Autodesk Inventor part; units mm, degrees
ref_plane "YZ Plane" through (0, 0, 0) normal (1, 0, 0) x (0, 1, 0)
ref_plane "XZ Plane" through (0, 0, 0) normal (0, 1, 0) x (-1, 0, 0)
ref_plane "XY Plane" through (0, 0, 0) normal (0, 0, 1) x (1, 0, 0)
sketch "Sketch2" plane through (0, 0, 0) normal (0, 1, 0) x (-1, 0, 0)
  line L0 (-12, 4) -> (12, 4)
  line L1 (12, 4) -> (12, -4)
  line L2 (12, -4) -> (-12, -4)
  line L3 (-12, -4) -> (-12, 4)
  point P0 (0, 0)
  point P1 (0, 4)
  point P2 (-12, 0)
  dimension "d0" = 24
  dimension "d1" = 8
extrude "Extrusion1" add sketch "Sketch2" along normal blind 3.2
sketch "Sketch3" plane through (0, 0, 0) normal (0, -1, 0) x (1, 0, 0)
  line L0 (12, 4) -> (-12, 4)
  line L1 (-12, 4) -> (-12, -4)
  line L2 (-10.4, 2.4) -> (10.4, 2.4)
  line L3 (10.4, 2.4) -> (10.4, -2.4)
  line L4 (10.4, -2.4) -> (-10.4, -2.4)
  line L5 (-10.4, -2.4) -> (-10.4, 2.4)
  circle A0 centre (-4, 4) radius 3.2569
  circle A1 centre (-4, 4) radius 2.4
  line L6 (-12, -4) -> (12, -4)
  circle A2 centre (-4, 0) radius 1.6
  line L7 (12, -4) -> (12, 4)
  line L8 (-8, 0) -> (0, 0) construction
  line L9 (0, 0) -> (8, 0) construction
  line L10 (-11.6, 3.6) -> (11.6, 3.6)
  line L11 (11.6, 3.6) -> (11.6, -3.6)
  line L12 (11.6, -3.6) -> (-11.6, -3.6)
  line L13 (-11.6, -3.6) -> (-11.6, 3.6)
  point P0 (-10.4, 0)
  point P1 (0, 2.4)
  point P2 (-4, 0)
  point P3 (0, 3.6)
  point P4 (-11.6, 0)
  dimension "d8" = 1.6
  dimension "d60" = 6.5137
  dimension "d61" = 4.8
  dimension "d62" = 1.6
  dimension "d75" = 8
  dimension "d76" = 8
  dimension "d86" = 3.2
  dimension "d89" = 8
  dimension "d95" = 0.4
  dimension "d96" = 0.4
extrude "Extrusion2" cut sketch "Sketch3" against normal blind 1.6 contours A0 A2 A1 L2 | L2 L3 L4 L5 A0 A2 | A1 L2 | L2 A1 A2 A0 | A2 A0 | A0 A2
extrude "Extrusion7" cut sketch "Sketch3" against normal blind 0.4 contours L7 L6 L1 L0 A0 L10 L13 L12 L11 | A0 L10 A1 L0 | A1 L10 L0 | L0 A1 L10 A0
fillet "Fillet1" radius 0.1 8 edges at (-12, 1.8, 4) (0, 3.2, 4) (-12, 3.2, 0) (0, 3.2, -4) (12, 3.2, 0) (12, 1.8, 4) (12, 1.8, -4) (-12, 1.8, -4)
sketch "Skizze10" plane through (0, 3.2, 0) normal (0, 1, 0) x (1, 0, 0)
  line L0 (-11.9, -3.9) -> (-11.9, 3.9)
  line L1 (-11.9, -3.9419) -> (-11.9, 3.9419) construction
  line L2 (-11.9, 3.9419) -> (11.9, 3.9419) construction
  line L3 (11.9, 3.9419) -> (11.9, -3.9419) construction
  line L4 (11.9, -3.9419) -> (-11.9, -3.9419) construction
  point P0 (0, 0)
  point P1 (0, 3.9419)
  point P2 (-11.9, 0)
  point P3 (-11.9, 0)
decal "Aufkleber1"
equation "\"d4\" = 0.333333 * lh"
equation "\"d8\" = d62"
equation "\"d60\" = tubeod"
equation "\"d61\" = kd"
equation "\"d62\" = wall"
equation "\"d75\" = lu"
equation "\"d76\" = d75"
equation "\"d86\" = pd"
equation "\"d89\" = lu"
equation "\"d95\" = gw"
equation "\"d96\" = gw"
equation "\"d11\" = 0.333333 * lh - topthk"
equation "\"d97\" = gh"
properties part number "42146_63864_1" material "ABS Plastic"
Could you check a few things on this model? Use its own coordinates, in mm. A direction names the side the tool comes from. Give positions to 0.01 mm unless a question says otherwise; leave off trailing zeros. Loops run counter-clockwise (first coordinate to the right, second up) from the corner with the lowest first, then second, coordinate; pieces in that order, holes last. Notation, with made-up numbers: (60.25, 16) -> (98.25, 16) arc R20 ccw to (98.25, 20) -> close; hole circle Ø10 at (13, 29). An arc over 180 degrees is marked (long way). Answer as CSV lines item,"result". Start each with the question number.
(1) I need wall thicknesses on probe 1 along Z at (x, y) = (-5.25, 0.5); probe 2 along X at (y, z) = (0.5, 0); probe 3 along Z at (x, y) = (4.25, 0.3). Which ranges of each line are inside material? Lowest first, please.
(2) If we section it at A-A on y = 0.65: Write out the boundary of the cut face in (x, z).
(3) Which directions (+Z, -Z, +X, -X, +Y, -Y) give clear straight access to the entire face, cutting with the end or side of a thin tool? Please do faces 4 (the flat face through (0, 1, -2.4)), 5 (the flat face through (12, 2, 0)).
(4) If we section it at C-C on x = 0: Write out the boundary of the cut face in (y, z), then the cut area to 3 significant figures.
(5) We'd pull the mould along X, two halves only. Please class faces 1 (the flat face through (10.4, 1, 0)), 2 (the flat face through (0, 3.2, 0)), 3 (the flat face through (-12, 2, 0)): released by +X, released by -X, zero draft, split by the parting line, or undercut.
(6) If we section it at B-B on z = -0.5: Write out the boundary of the cut face in (x, y).
(7) I'm going to push a flat-ended pin straight in: pin 1 Ø2.5 at (x, z) = (2.5, 0) entering from -Y. Where does the tip first touch, or does it pass through?
Computed:
1,probe 1,"z = -4 to -2.4, 2.4 to 4"
1,probe 2,"x = -12 to -10.4, 10.4 to 12"
1,probe 3,"z = -3.6 to -2.4, 2.4 to 3.6"
2,outline,"(-12, -3.9) arc R0.1 ccw to (-11.9, -4) -> (11.9, -4) arc R0.1 ccw to (12, -3.9) -> (12, 3.9) arc R0.1 ccw to (11.9, 4) -> (-11.9, 4) arc R0.1 ccw to (-12, 3.9) -> close; hole (-10.4, -2.4) -> (10.4, -2.4) -> (10.4, 2.4) -> (-10.4, 2.4) -> close"
3,face 4,"-Y"
3,face 5,"+Z, -Z, +X, +Y, -Y"
4,outline,"(0, -3.6) -> (0.4, -3.6) -> (0.4, -4) -> (3.1, -4) arc R0.1 ccw to (3.2, -3.9) -> (3.2, 3.9) arc R0.1 ccw to (3.1, 4) -> (0.4, 4) -> (0.4, 3.6) -> (0, 3.6) -> (0, 2.4) -> (1.6, 2.4) -> (1.6, -2.4) -> (0, -2.4) -> close"
4,area,"17.6 mm2"
5,face 1,"undercut"
5,face 2,"zero draft"
5,face 3,"released by -X"
6,outline,"(-12, 0.4) -> (-11.6, 0.4) -> (-11.6, 0) -> (-10.4, 0) -> (-10.4, 1.6) -> (10.4, 1.6) -> (10.4, 0) -> (11.6, 0) -> (11.6, 0.4) -> (12, 0.4) -> (12, 3.1) arc R0.1 ccw to (11.9, 3.2) -> (-11.9, 3.2) arc R0.1 ccw to (-12, 3.1) -> close"
7,pin 1,"stops at y = 1.6"
